Input: part model. Units: mm. Frame: model coordinates. A direction names the side the tool comes from. Coordinates: 2 decimals unless noted, no trailing zeros. Order: outer loops, then holes, each group sorted by start corner. A loop starts at its lowest first (then second) coordinate and runs counter-clockwise, first axis right, second up. Notation, with made-up numbers: (70.5, 32) -> (111.5, 32) arc R29 cw to (111.5, 54) -> close; hole circle Ø5 at (32, 86). An arc over 180 degrees is marked (long way). One line per question, with ' | ' between items.
```python
from build123d import *

# Parameters (mm, degrees)
CUT_EXTRUDE1_DEPTH              = 18.0086
CUT_EXTRUDE2_DEPTH              = 2.032
TAP_DRILL_FOR_M4X0_7_TAP2_D     = 3.3
TAP_DRILL_FOR_M4X0_7_TAP2_DEPTH = 12.7
SKETCH8_W                       = 8.89
SKETCH8_H                       = 4.826
BOSS_EXTRUDE1_DEPTH             = 0.254


with BuildPart() as part:
    # Sketch1 → Revolve1 (revolve)
    with BuildSketch(Plane.XY):
        Polygon((0, 0), (0, 3.81), (5.08, 3.81), (5.08, 11.43), (9.017, 11.43), (9.017, 20.955), (31.115, 20.955), (31.115, 22.2504), (69.215, 22.2504), (69.215, 20.955), (75.565, 20.955), (75.565, 22.5044), (132.08, 22.5044), (132.08, 12.954), (134.112, 12.954), (134.112, 4.99999), (159.004, 4.99999), (159.004, 0), align=None)
    revolve(axis=Axis((0, 0, 0), (1, 0, 0)))

    # Sketch2 → Cut-Extrude1 (cut)
    with BuildSketch(Plane(origin=(159.004, 0, 0), x_dir=(0, 0, -1), z_dir=(1, 0, 0))):
        with BuildLine():
            Line((-1.9939, -4.585222218), (-1.9939, -2.553222218))
            Line((-1.9939, -2.553222218), (1.9939, -2.553222218))
            Line((1.9939, -2.553222218), (1.9939, -4.585222218))
            ThreePointArc((1.9939, -4.585222218), (0, -4.99999), (-1.9939, -4.585222218))
        make_face()
    extrude(amount=-CUT_EXTRUDE1_DEPTH, mode=Mode.SUBTRACT)

    # Sketch3 → Cut-Extrude2 (cut)
    with BuildSketch(Plane(origin=(134.112, 0, 0), x_dir=(0, 0, -1), z_dir=(1, 0, 0))):
        with BuildLine():
            Line((-4.875460363, 12.0015), (4.875460363, 12.0015))
            ThreePointArc((4.875460363, 12.0015), (0, 12.954), (-4.875460363, 12.0015))
        make_face()
        with BuildLine():
            Line((-4.875460363, -12.0015), (4.875460363, -12.0015))
            ThreePointArc((4.875460363, -12.0015), (0, -12.954), (-4.875460363, -12.0015))
        make_face()
    extrude(amount=-CUT_EXTRUDE2_DEPTH, mode=Mode.SUBTRACT)

    # Tap Drill for M4x0.7 Tap2
    with Locations(Plane(origin=(132.08, 0, 0), x_dir=(0, 0, -1), z_dir=(1, 0, 0))):
        with Locations((-12.374792935, 12.374792935), (12.374792935, -12.374792935), (12.374792935, 12.374792935), (-12.374792935, -12.374792935)):
            Hole(TAP_DRILL_FOR_M4X0_7_TAP2_D / 2, depth=TAP_DRILL_FOR_M4X0_7_TAP2_DEPTH)

    # Sketch8 → Boss-Extrude1 (add, symmetric)
    with BuildSketch(Plane.XY.offset(19.05)):
        with Locations((4.572, 0)):
            Rectangle(SKETCH8_W, SKETCH8_H)
    boss_extrude1 = extrude(amount=BOSS_EXTRUDE1_DEPTH, both=True)

    # Mirror1: Boss-Extrude1 across plane
    add(boss_extrude1.mirror(Plane.XY))


solid = part.part
```
1. Mould query, pull axis Y, two halves, no side actions, for faces 1 (the face through (5.08, 3, 3)), 2 (the face through (50.432, 21.223, 6.683)), 3 (the face through (119.38, 12, 12)). Classes: released by +Y, released by -Y, zero draft, split by the parting line, or undercut.
Recorded:
face 1: zero draft | face 2: split by the parting line | face 3: undercut
2. Access query for faces 4 (the face through (132.08, 10, -10)), 5 (the face through (7.076, 10.902, 3.433)), 6 (the face through (5, 0, 19.304)). Directions: +Z, -Z, +X, -X, +Y, -Y. A direction counts if a zero-diameter tool reaches every point of the face in a straight line with its end or side. Return the directions, or none.
Recorded:
face 4: +X | face 5: -X | face 6: +Z, -X, +Y, -Y
3. Pin query (flat end, axial travel): pin 1 Ø1.7 at (y, z) = (12, -12) entering from +X; pin 2 Ø1 at (x, z) = (133.5, 1) entering from -Y; pin 3 Ø3.5 at (y, z) = (12.5, 11.5) entering from +X. Return the tip coordinate at first contact, or that it passes through.
Recorded:
pin 1: stops at x = 119.38 | pin 2: stops at y = -12 | pin 3: stops at x = 132.08
4. Cut plane C-C, the plane x = 101.5. Return loops of the section in (y, z), and give its area (3 significant figures).
Recorded:
outline: circle Ø45.01 at (0, 0) | area: 1,590 mm^2
5. Cut plane D-D, the plane z = 17. Return loops of the section in (x, y) (1 decimal), and give its area (3 significant figures).
Recorded:
outline: (9, -12.3) -> (31.1, -12.3) -> (31.1, -14.4) -> (69.2, -14.4) -> (69.2, -12.3) -> (75.6, -12.3) -> (75.6, -14.7) -> (132.1, -14.7) -> (132.1, 14.7) -> (75.6, 14.7) -> (75.6, 12.3) -> (69.2, 12.3) -> (69.2, 14.4) -> (31.1, 14.4) -> (31.1, 12.3) -> (9, 12.3) -> close | area: 3,460 mm^2
6. Cut plane B-B, the plane y = 7. Return loops of the section in (x, z) (3 decimals), and give its area (3 significant figures).
Recorded:
outline: (5.08, -9.036) -> (9.017, -9.036) -> (9.017, -19.751) -> (31.115, -19.751) -> (31.115, -21.121) -> (69.215, -21.121) -> (69.215, -19.751) -> (75.565, -19.751) -> (75.565, -21.388) -> (132.08, -21.388) -> (132.08, -10.9) -> (134.112, -10.9) -> (134.112, 10.9) -> (132.08, 10.9) -> (132.08, 21.388) -> (75.565, 21.388) -> (75.565, 19.751) -> (69.215, 19.751) -> (69.215, 21.121) -> (31.115, 21.121) -> (31.115, 19.751) -> (9.017, 19.751) -> (9.017, 9.036) -> (5.08, 9.036) -> close | area: 5,270 mm^2
7. Ray query, line 1 (X direction, y = 19, z = 9.5) (3 decimals); line 2 (X direction, y = -1, z = 13); line 3 (X direction, y = -13, z = 12). Return the intervals inside material, ascending. Write a range as [from, to].
Recorded:
line 1: x = [31.115, 69.215], [75.565, 132.08] | line 2: x = [9.02, 132.08] | line 3: x = [9.02, 119.38]
